Could you check a few things on this model? Use its own coordinates, in mm. A direction names the side the tool comes from. Give positions to 0.01 mm unless a question says otherwise; leave off trailing zeros. Order: outer loops, then holes, each group sorted by start corner. A loop starts at its lowest first (then second) coordinate and runs counter-clockwise, first axis right, second up. Notation, with made-up numbers: (52.25, 73) -> (107.25, 73) arc R19 cw to (107.25, 77) -> close; hole circle Ø8 at (28, -7.75). An arc over 180 degrees is marked (long way). Use one line per item in the form item = value. Start each with the question number.
Autodesk Inventor part; units mm, degrees
ref_plane "YZ Plane" through (0, 0, 0) normal (1, 0, 0) x (0, 1, 0)
ref_plane "XZ Plane" through (0, 0, 0) normal (0, 1, 0) x (-1, 0, 0)
ref_plane "XY Plane" through (0, 0, 0) normal (0, 0, 1) x (1, 0, 0)
sketch "Sketch1" plane through (0, 0, 0) normal (0, 0, 1) x (1, 0, 0)
  line L0 (0, 0) -> (0, 6.35)
  line L1 (0, 0) -> (7.9375, 0)
  line L2 (7.9375, 0) -> (8.1915, 0)
  line L3 (0, 6.35) -> (7.9375, 6.35) construction
  line L4 (7.9375, 6.35) -> (7.9375, 0) construction
  line L5 (0, 5.5563) -> (7.9375, 5.5563) construction
  line L6 (7.9375, 6.35) -> (7.9375, 7.9375) construction
  line L7 (7.9375, 7.9375) -> (34.2265, 7.9375) construction
  line L8 (34.2265, 0) -> (34.2265, 7.9375) construction
  line L9 (34.2265, 7.3323) -> (37.4015, 7.3323) construction
  line L10 (37.4015, 7.3323) -> (37.4015, 0) construction
  line L11 (37.4015, 0) -> (34.2265, 0)
  line L12 (37.4015, 6.35) -> (45.593, 6.35) construction
  line L13 (45.593, 6.35) -> (45.593, 0) construction
  line L14 (37.4015, 0) -> (37.6555, 0)
  line L15 (37.6555, 0) -> (45.593, 0)
  line L16 (37.6555, 0) -> (37.6555, 6.35) construction
  line L17 (7.9375, 5.5563) -> (45.593, 5.5563) construction
  line L18 (16.4059, 7.874) -> (17.6759, 7.874) construction
  line L19 (0, 3.1115) -> (26.9557, 3.1115)
  line L20 (0, 5.1753) -> (45.593, 5.1753)
  line L21 (8.1915, 0) -> (8.1915, 7.9375) construction
  line L22 (8.1915, 0) -> (8.9852, 0)
  line L23 (8.9852, 0) -> (8.9852, 7.9375) construction
  line L24 (8.9852, 7.9375) -> (8.9852, 25.0214) construction
  line L25 (8.9852, 25.0214) -> (13.7477, 25.0214) construction
  line L26 (13.7477, 25.0214) -> (13.7477, 0) construction
  line L27 (13.7477, 0) -> (8.9852, 0)
  line L28 (13.7477, 17.4625) -> (21.082, 17.4625) construction
  line L29 (13.7477, 25.0214) -> (18.5102, 25.0214) construction
  line L30 (18.5102, 25.0214) -> (18.5103, 0) construction
  line L31 (18.5103, 0) -> (13.7477, 0)
  line L32 (21.082, 17.4625) -> (21.082, 0) construction
  line L33 (21.082, 0) -> (18.5103, 0)
  line L34 (21.082, 0) -> (21.8758, 0)
  line L35 (21.8758, 0) -> (21.8758, 14.2875) construction
  line L36 (21.8758, 14.2875) -> (21.082, 14.2875) construction
  line L37 (8.1915, 7.9375) -> (8.1915, 14.2875) construction
  line L38 (8.1915, 14.2875) -> (8.9852, 14.2875) construction
  line L39 (21.8758, 30.0415) -> (26.6382, 30.0415) construction
  line L40 (26.6382, 30.0415) -> (26.6382, 0) construction
  line L41 (26.6382, 0) -> (21.8758, 0)
  line L42 (26.6382, 30.0415) -> (31.4007, 30.0415) construction
  line L43 (31.4007, 30.0415) -> (31.4007, 0) construction
  line L44 (26.6382, 0) -> (31.4007, 0)
  line L45 (26.6382, 17.4625) -> (33.9725, 17.4625) construction
  line L46 (33.9725, 17.4625) -> (33.9725, 0) construction
  line L47 (33.9725, 0) -> (31.4007, 0)
  line L48 (21.8758, 14.2875) -> (21.8758, 30.0415) construction
  line L49 (33.9725, 0) -> (34.2265, 0)
  line L50 (11.3665, 25.0214) -> (11.3665, 0) construction
  line L51 (24.257, 30.0415) -> (24.257, 0) construction
  circle A0 centre (11.3665, 7.5565) radius 2.3813 construction
  circle A1 centre (11.3665, 5.4927) radius 2.3813 construction
  line L52 (8.9893, 7.874) -> (10.2593, 7.874) construction
  circle A2 centre (24.257, 5.4927) radius 2.3812 construction
  circle A3 centre (24.257, 7.5565) radius 2.3812 construction
  line L53 (23.0177, 7.874) -> (24.0459, 7.874) construction
  line L54 (14.6367, 5.1752) -> (12.573, 3.1115) construction
  line L55 (20.9867, 5.1752) -> (23.0505, 3.1115) construction
  line L56 (10.7315, 5.1752) -> (8.6677, 3.1115) construction
  line L57 (10.4775, 5.1752) -> (8.4137, 3.1115) construction
  line L58 (0, 3.5719) -> (8.8741, 3.5719) construction
  line L59 (0, 3.5719) -> (-1.5875, 3.5719) construction
  line L60 (-1.5875, 3.5719) -> (-1.5875, 6.35) construction
  line L61 (-1.5875, 6.35) -> (0, 6.35) construction
  line L62 (26.7144, 7.9375) -> (26.7144, 0) construction
  line L63 (24.892, 5.1752) -> (26.9557, 3.1115)
  line L64 (26.7144, 5.5563) -> (28.1834, 3.1115) construction
  line L65 (16.8275, 5.1752) -> (18.8912, 3.1115) construction
  line L66 (37.5179, 3.1115) -> (37.5179, 0) construction
  line L67 (16.4782, 3.1115) -> (18.542, 5.1752)
  line L68 (69.3538, 20.0694) -> (73.1082, 25.272) construction
  line L69 (73.1082, 25.272) -> (79.491, 24.6219) construction
  line L70 (79.491, 24.6219) -> (82.1194, 18.7692) construction
  line L71 (82.1194, 18.7692) -> (78.365, 13.5666) construction
  line L72 (78.365, 13.5666) -> (71.9822, 14.2167) construction
  line L73 (71.9822, 14.2167) -> (69.3538, 20.0694) construction
  circle A4 centre (75.7366, 19.4193) radius 6.4158 construction
  line L74 (45.593, 5.5563) -> (53.7803, 5.5563) construction
  line L75 (53.7803, 5.5563) -> (53.7803, 0) construction
  line L76 (53.7803, 0) -> (45.593, 0) construction
  line L77 (28.026, 3.3734) -> (45.593, 3.3734) construction
  line L78 (31.323, 0) -> (29.4534, 3.1115)
  line L79 (37.5179, 3.1115) -> (39.3875, 0)
  line L80 (37.7719, 3.1115) -> (39.6415, 0) construction
  line L81 (8.909, 7.9375) -> (8.909, 0) construction
  line L82 (37.7719, 3.1115) -> (37.6145, 3.3734) construction
  line L83 (37.5179, 3.1115) -> (45.593, 3.1115) construction
  line L84 (26.9557, 3.1115) -> (37.5179, 3.1115)
  line L85 (0, 0) -> (-1.5875, 0)
  line L86 (-1.5875, 0) -> (-1.5875, 3.1115)
  line L87 (-1.5875, 3.1115) -> (0, 3.1115)
  line L88 (-1.5875, 0) -> (-2.3812, 0)
  line L89 (-2.3812, 0) -> (-2.3813, 3.1115)
  line L90 (-2.3813, 3.1115) -> (-1.5875, 3.1115)
  point P0 (11.3665, 3.1115)
  point P1 (11.3665, 5.1752)
  point P2 (24.257, 5.1752)
  dimension "d78" = 4.7625
  dimension "d82" = 4.7625
  dimension "d116" = 12.8316
  dimension "d40" = 0.254
  dimension "d41" = 7.9375
  dimension "d42" = 6.35
  dimension "d43" = 5.5563
  dimension "d44" = 7.9375
  dimension "d46" = 7.3323
  dimension "d47" = 3.175
  dimension "d48" = 0.254
  dimension "d49" = 6.35
  dimension "d50" = 7.9375
  dimension "d53" = 1.27
  dimension "d54" = 0.0635
  dimension "d58" = 3.1115
  dimension "d61" = 5.1753
  dimension "d63" = 0.7937
  dimension "d64" = 4.7625
  dimension "d65" = 7.3342
  dimension "d66" = 17.4625
  dimension "d67" = 4.7625
  dimension "d68" = 0.7937
  dimension "d69" = 14.2875
  dimension "d70" = 14.2875
  dimension "d71" = 4.7625
  dimension "d72" = 4.7625
  dimension "d73" = 7.3342
  dimension "d74" = 17.4625
  dimension "d75" = 0.254
  dimension "d76" = 12.8905
  dimension "d77" = 0.381
  dimension "d80" = 0.0635
  dimension "d81" = 4.7625
  dimension "d83" = 0.381
  dimension "d84" = 0.0635
  dimension "d85" = 45
  dimension "d86" = 45
  dimension "d88" = 1.2065
  dimension "d89" = 6.35
  dimension "d90" = 3.2702
  dimension "d91" = 0.635
  dimension "d92" = 45
  dimension "d93" = 0.254
  dimension "d94" = 3.5719
  dimension "d95" = 0.4604
  dimension "d96" = 1.5875
  dimension "d97" = 2.7781
  dimension "d98" = 1.6034
  dimension "d99" = 3.9053
  dimension "d101" = 3.2702
  dimension "d102" = 4.9149
  dimension "d103" = 0.635
  dimension "d105" = 59
  dimension "d106" = 2.4977
  dimension "d107" = 6.35
  dimension "d108" = 45
  dimension "d109" = 8.0645
  dimension "d110" = 10.5622
  dimension "d114" = 6.35
  dimension "d115" = 11.1125
  dimension "d117" = 5.5563
  dimension "d118" = 3.1115
  dimension "d120" = 3.3734
  dimension "d121" = 59
  dimension "d122" = 1.27
  dimension "d123" = 59
revolve "Revolution1" add sketch "Sketch1" angle 360 about axis through (21.082, 0, 0) along (-1, 0, 0) contours L85 L86 L87 L0 | L0 L19 L84 L78 L44 L41 L34 L33 L31 L27 L22 L2 L1 | L88 L89 L90 L86 | L67 L20 L63 L19 | L84 L79 L15 L14 L11 L49 L47 L44 L78
fillet "Fillet1" radius 0.381 3 edges at (18.542, -5.1752, 0) (24.892, -5.1752, 0) (26.9557, -3.1115, 0)
sketch "Sketch12" plane through (-2.3812, 0, 0) normal (-1, 0, 0) x (0, 0, 1)
  circle A0 centre (0, 0) radius 3.1115
  circle A1 centre (0, 0) radius 2.3812
  circle A2 centre (0, 0) radius 3.1115
  dimension "d160" = 4.7625
extrude "Extrusion11" add sketch "Sketch12" along normal blind 6.8199 contours A1
sketch "Sketch13" plane through (0, 0, 0) normal (0, 1, 0) x (-1, 0, 0)
  line L0 (9.2011, -2.3812) -> (9.2011, 2.3812)
  circle A0 centre (8.1471, 0) radius 0.7874
  line L1 (0, 0) -> (8.1471, 0) construction
  line L2 (2.3813, 3.1115) -> (2.3813, -3.1115)
  point P0 (7.3597, 0)
  dimension "d164" = 1.5748
  dimension "d169" = 4.9784
extrude "Extrusion12" cut sketch "Sketch13" along normal through all both and the other way through all
ref_plane "Work Plane2" through (-1.5875, 0, 0) normal (-1, 0, 0) x (0, 0, 1)
properties part number "Ball Shisting Shaft Outline Sketch"
(1) Imagine slicing it at B-B (x = 22.5). Write out the boundary of the cut face in (y, z).
(2) Please list where these lines run through material, in increasing order: probe 1 along Y at (x, z) = (-2, -0.25); probe 2 along X at (y, z) = (0.45, 0).
(3) We'd pull the mould along Z, two halves only. Please class faces 4 (the flat face through (-9.201, 0, 0)), 5 (the cylindrical face through (-7.522, 0.033, -0.479)), 6 (the conical face through (39.06, -0.12, 0.53)): pulls with the +Z half, pulls with the -Z half, needs draft (parallel to the pull), parting line crosses it, or undercut.
(4) Which directions (+Z, -Z, +X, -X, +Y, -Y) give clear straight access to the entire face, cutting with the end or side of a thin tool? Please do faces 1 (the cylindrical face through (32.39, -0.67, -3.04)), 2 (the cylindrical face through (21.76, 2.39, -4.59)), 3 (the cylindrical face through (7.18, -0.67, -3.04)).
(5) Imagine slicing it at A-A (x = 35). Write out the boundary of the cut face in (y, z), plus the area to 3 significant figures.
(6) I'm going to push flat-ended pins straight in: pin 1 Ø2 at (x, y) = (15, 2) entering from +Z; pin 2 Ø5 at (x, y) = (25.5, 3.5) entering from -Z; pin 3 Ø4 at (x, y) = (8.5, 3) entering from -Z. Where does each tip first touch, or does it pass through?
Calculated:
q1.outline = circle Ø10.35 at (0, 0)
q2.probe_1 = -3.1 to 3.1
q2.probe_2 = -9.2 to -8.93, -7.36 to 39.12
q3.face_4 = needs draft
q3.face_5 = undercut
q3.face_6 = parting line crosses it
q4.face_1 = +X
q4.face_2 = +X, -X
q4.face_3 = -X
q5.outline = circle Ø6.22 at (0, 0)
q5.area = 30.4 mm2
q6.pin_1 = 2.95
q6.pin_2 = -5.05
q6.pin_3 = -2.95
